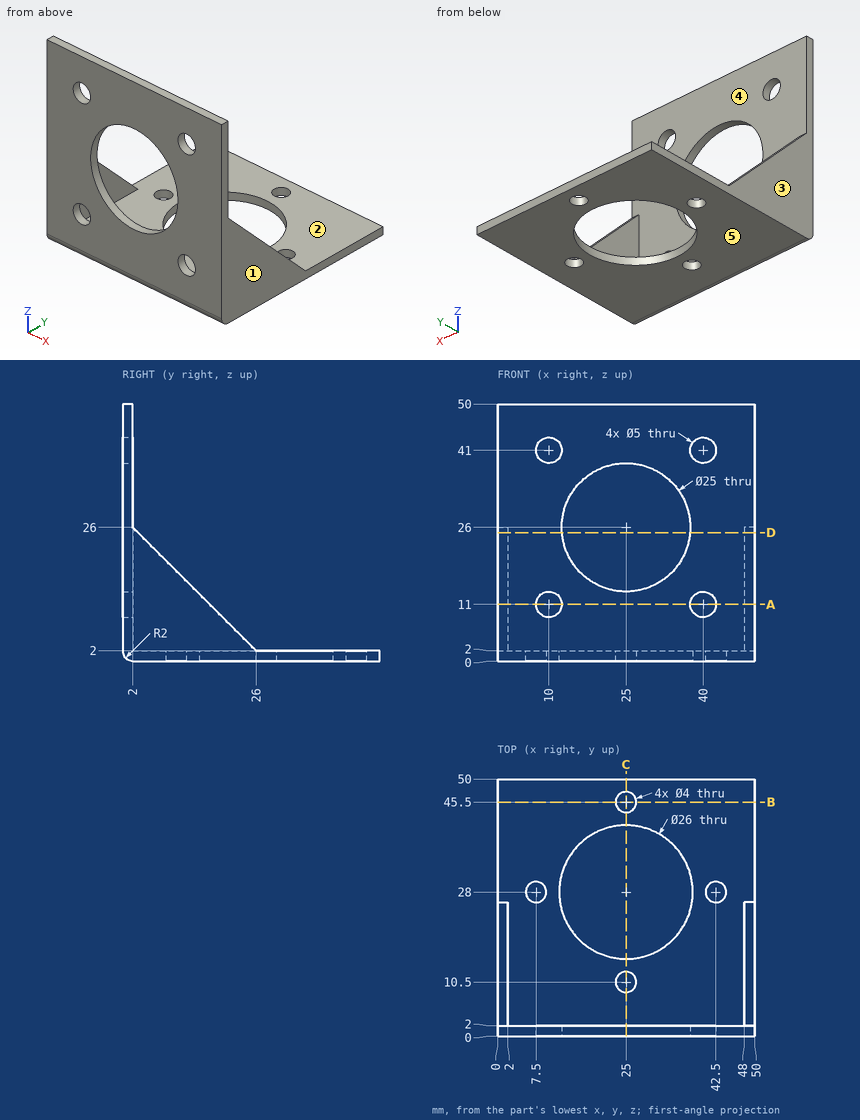
Could you check a few things on this drawing? It's one solid part, dimensions in mm from its lowest x, y, z. A direction names the side the tool comes from. Coordinates: 2 decimals unless noted, no trailing zeros. Write each loop counter-clockwise with the first axis right and the second up, starting at its lowest first coordinate (ties: lowest second). Pieces come first, ordered by that corner, then holes. Notation, with made-up numbers: (2, -12) - (36, -12) arc R23 ccw to (36, 27) - close; hole circle Ø7 at (-13.5, 12.25). An arc over 180 degrees is marked (long way). Return JSON: item names as keys, results as strings. Group by question number.
Item 1: Which directions (+Z, -Z, +X, -X, +Y, -Y) give clear straight access to the entire face, cutting with the end or side of a thin tool? Please do the marked faces 4 and 5.
Item 2: If we section it at C-C (x = 25): Write out the boundary of the cut face in (y, z).
Item 3: I'm going to push flat-ended pins straight in: pin 1 Ø8 at (x, z) = (10, 11) entering from +Y; pin 2 Ø4.5 at (x, y) = (42.5, 28) entering from +Z. Where does each tip first touch, or does it pass through?
Item 4: Please list where these lines run through material, in increasing order: probe 1 along X at (y, z) = (0.9, 41); probe 2 along Y at (x, z) = (10.5, 22).
Item 5: If we section it at B-B (y = 45.5): Write out the boundary of the cut face in (x, z).
Item 6: If we section it at D-D (z = 25): Write out the boundary of the cut face in (x, y).
Item 7: We'd pull the mould along X, two halves only. Please class the marked faces 1, 2 and 3: pulls with the +X half, pulls with the -X half, needs draft (parallel to the pull), parting line crosses it, or undercut.
Item 8: If we section it at A-A (z = 11): Write out the boundary of the cut face in (x, y).
Return value:
{
 "1": {"face 4": "+Z, +Y", "face 5": "-Z, +X, -X, +Y, -Y"},
 "2": {"outline": "(0, 2) arc R2 ccw to (2, 0) - (8.5, 0) - (8.5, 2) - (2, 2) - (2, 13.5) - (0, 13.5) - close; (0, 38.5) - (2, 38.5) - (2, 50) - (0, 50) - close; (12.5, 0) - (15, 0) - (15, 2) - (12.5, 2) - close; (41, 0) - (43.5, 0) - (43.5, 2) - (41, 2) - close; (47.5, 0) - (50, 0) - (50, 2) - (47.5, 2) - close"},
 "3": {"pin 1": "stops at y = 2", "pin 2": "stops at z = 2"},
 "4": {"probe 1": "x = 0 to 7.5, 12.5 to 37.5, 42.5 to 50", "probe 2": "y = 0 to 2"},
 "5": {"outline": "(0, 0) - (23, 0) - (23, 2) - (0, 2) - close; (27, 0) - (50, 0) - (50, 2) - (27, 2) - close"},
 "6": {"outline": "(0, 0) - (12.54, 0) - (12.54, 2) - (2, 2) - (2, 3) - (0, 3) - close; (37.46, 0) - (50, 0) - (50, 3) - (48, 3) - (48, 2) - (37.46, 2) - close"},
 "7": {"face 1": "pulls with the +X half", "face 2": "undercut", "face 3": "pulls with the -X half"},
 "8": {"outline": "(0, 0) - (7.5, 0) - (7.5, 2) - (2, 2) - (2, 17) - (0, 17) - close; (12.5, 0) - (37.5, 0) - (37.5, 2) - (12.5, 2) - close; (42.5, 0) - (50, 0) - (50, 17) - (48, 17) - (48, 2) - (42.5, 2) - close"}
}
